```python
from build123d import *

# Parameters (mm, degrees)
BOSS_EXTRU_1_DEPTH           = 40
ENL_V_MAT_EXTRU_1_DEPTH      = 76.498344353
ENL_V_MAT_EXTRU_1_DEPTH_BACK = 76.498344353
ESQUISSE2_R                  = 2.25
ENL_V_MAT_EXTRU_2_DEPTH      = 76.498344353
ENL_V_MAT_EXTRU_2_DEPTH_BACK = 76.498344353
ESQUISSE3_R                  = 2.25
ENL_V_MAT_EXTRU_3_DEPTH      = 96.640449297
ENL_V_MAT_EXTRU_3_DEPTH_BACK = 20
ESQUISSE4_R                  = 2.1
BOSS_EXTRU_2_DEPTH           = 4
BOSS_EXTRU_3_START           = -40
BOSS_EXTRU_3_DEPTH           = 4
BOSS_EXTRU_4_DEPTH           = 3
BOSS_EXTRU_4_DEPTH_BACK      = 3
BOSS_EXTRU_4_START           = -20
CONG_1_R                     = 4


with BuildPart() as part:
    # Esquisse1 → Boss.-Extru.1 (new body)
    with BuildSketch(Plane(origin=(0, 0, 0), x_dir=(0, 0, -1), z_dir=(1, 0, 0))):
        Polygon((0, 0), (40, 0), (40, 10), (0, 10), (0, 36), (-15, 36), (-35, 1.358983849), (-20, -7.301270189), (-10, -7.301270189), (-10, -40), (0, -40), align=None)
    extrude(amount=BOSS_EXTRU_1_DEPTH)

    # Esquisse2 → Enlèv. mat.-Extru.1 (cut, two sides: drawn at the far end of the back side and taken through both)
    with BuildSketch(Plane(origin=(0, 10, 0), x_dir=(1, 0, 0), z_dir=(0, 1, 0)).offset(-ENL_V_MAT_EXTRU_1_DEPTH_BACK)):
        with Locations(Location((10, 30, 0), (0, 0, 270))):
            Circle(ESQUISSE2_R)
        with Locations(Location((30, 30, 0), (0, 0, 270))):
            Circle(ESQUISSE2_R)
        with Locations(Location((30, 10, 0), (0, 0, 270))):
            Circle(ESQUISSE2_R)
        with Locations(Location((10, 10, 0), (0, 0, 270))):
            Circle(ESQUISSE2_R)
    extrude(amount=ENL_V_MAT_EXTRU_1_DEPTH + ENL_V_MAT_EXTRU_1_DEPTH_BACK, mode=Mode.SUBTRACT)

    # Esquisse3 → Enlèv. mat.-Extru.2 (cut, two sides: drawn at the far end of the back side and taken through both)
    with BuildSketch(Plane.XY.offset(10).offset(-ENL_V_MAT_EXTRU_2_DEPTH_BACK)):
        with Locations((10, -33.650635095)):
            Circle(ESQUISSE3_R)
        with Locations((30, -33.650635095)):
            Circle(ESQUISSE3_R)
        with Locations((30, -13.650635095)):
            Circle(ESQUISSE3_R)
        with Locations((10, -13.650635095)):
            Circle(ESQUISSE3_R)
    extrude(amount=ENL_V_MAT_EXTRU_2_DEPTH + ENL_V_MAT_EXTRU_2_DEPTH_BACK, mode=Mode.SUBTRACT)

    # Esquisse4 → Enlèv. mat.-Extru.3 (cut, two sides: drawn at the far end of the back side and taken through both)
    with BuildSketch(Plane(origin=(0, 15.495190528, 26.838457268), x_dir=(1, 0, 0), z_dir=(0, 0.4999999999999946, 0.8660254037844419)).offset(-ENL_V_MAT_EXTRU_3_DEPTH_BACK)):
        with Locations(Location((20, 13.676914536, 0), (0, 0, 90))):
            Circle(ESQUISSE4_R)
        with Locations(Location((20, -6.323085464, 0), (0, 0, 90))):
            Circle(ESQUISSE4_R)
    extrude(amount=ENL_V_MAT_EXTRU_3_DEPTH + ENL_V_MAT_EXTRU_3_DEPTH_BACK, mode=Mode.SUBTRACT)

    # Esquisse5 → Boss.-Extru.2 (add)
    with BuildSketch(Plane(origin=(40, 0, 0), x_dir=(0, 0, -1), z_dir=(1, 0, 0))):
        Polygon((40, 10), (0, 36), (0, 10), align=None)
    extrude(amount=-BOSS_EXTRU_2_DEPTH)

    # Esquisse5<2> → Boss.-Extru.3 (add)
    with BuildSketch(Plane(origin=(40, 0, 0), x_dir=(0, 0, -1), z_dir=(1, 0, 0)).offset(BOSS_EXTRU_3_START)):
        Polygon((40, 10), (0, 36), (0, 10), align=None)
    extrude(amount=BOSS_EXTRU_3_DEPTH)

    # Esquisse5<3> → Boss.-Extru.4 (add, two sides: drawn at the far end of the back side and taken through both)
    with BuildSketch(Plane(origin=(40, 0, 0), x_dir=(0, 0, -1), z_dir=(1, 0, 0)).offset(BOSS_EXTRU_4_START - BOSS_EXTRU_4_DEPTH_BACK)):
        Polygon((40, 10), (0, 36), (0, 10), align=None)
    extrude(amount=BOSS_EXTRU_4_DEPTH + BOSS_EXTRU_4_DEPTH_BACK)

    # Congé1
    cong_1_edges = [part.edges().sort_by_distance(p)[0] for p in [
        (0, 5, -40),
        (40, 5, -40),
        (0, -40, 5),
        (40, -40, 5),
    ]]
    fillet(cong_1_edges, radius=CONG_1_R)


solid = part.part
```
Verification items for the finished model (mm, model axes). A direction names the side the tool comes from. Round coordinates to 2 decimals unless told otherwise and drop trailing zeros. Write each loop counter-clockwise with the first axis right and the second up, starting at its lowest first coordinate (ties: lowest second). Pieces come first, ordered by that corner, then holes. Notation, with made-up numbers: (18, -26.75) -> (67, -26.75) arc R26 ccw to (67, 4.25) -> close; hole circle Ø5 at (83.5, 65). An arc over 180 degrees is marked (long way). Write each question's results on one line, items separated by ' | '.
Q1. Sectioned sample at A-A, the plane z = -30. Record the boundary of the cut face in (x, y).
Derived:
outline: (0, 0) -> (7.75, 0) -> (7.75, 10) -> (4, 10) -> (4, 16.5) -> (0, 16.5) -> close; (12.25, 0) -> (27.75, 0) -> (27.75, 10) -> (23, 10) -> (23, 16.5) -> (17, 16.5) -> (17, 10) -> (12.25, 10) -> close; (32.25, 0) -> (40, 0) -> (40, 16.5) -> (36, 16.5) -> (36, 10) -> (32.25, 10) -> close
Q2. Sectioned sample at D-D, the plane y = -18.5. Record the boundary of the cut face in (x, z), and give its area (3 significant figures).
Derived:
outline: (0, 0) -> (40, 0) -> (40, 10) -> (0, 10) -> close | area: 400 mm²
Q3. Sectioned sample at C-C, the plane z = -2. Record the boundary of the cut face in (x, y), and give its area (3 significant figures).
Derived:
outline: (0, 0) -> (40, 0) -> (40, 34.7) -> (36, 34.7) -> (36, 10) -> (23, 10) -> (23, 34.7) -> (17, 34.7) -> (17, 10) -> (4, 10) -> (4, 34.7) -> (0, 34.7) -> close | area: 746 mm²
Q4. Thickness scan on probe 1 along Y at (x, z) = (10, 6); probe 2 along X at (y, z) = (3.25, -30); probe 3 along X at (y, z) = (-15, 8.5). Record the ranges inside material, lowest first.
Derived:
probe 1: y = -40 to -35.9, -31.4 to -15.9, -11.4 to 36 | probe 2: x = 0 to 7.75, 12.25 to 27.75, 32.25 to 40 | probe 3: x = 0 to 8.2, 11.8 to 28.2, 31.8 to 40
Q5. Access from +Z, -Z, +X, -X, +Y, -Y to the whole of each face (thin tool, end or side, straight path). Record for faces 1 (the face through (30.099, 4.93, -12.248)), 2 (the face through (29, 23, 0)), 3 (the face through (20, -23, 10)).
Derived:
face 1: +Y, -Y | face 2: -Z, +Y | face 3: +Z, +X, -X, -Y
Q6. Draft check along X on faces 4 (the face through (11.52, 4.93, -11.66)), 5 (the face through (0, 9, 0)), 6 (the face through (2, 23, -20)). Enter one of: released by +X, released by -X, zero draft, split by the parting line, or undercut.
Derived:
face 4: undercut | face 5: released by -X | face 6: zero draft
Q7. Go/stop test with flat-tipped pins: pin 1 Ø7 at (x, y) = (10, -13.65) entering from -Z; pin 2 Ø10 at (x, y) = (28, -3.5) entering from +Z; pin 3 Ø2 at (x, y) = (17, 3) entering from +Z; pin 4 Ø4 at (y, z) = (21, 5) entering from -X. Record where each tip stops, or that it passes through.
Derived:
pin 1: stops at z = 0 | pin 2: stops at z = 35 | pin 3: stops at z = 34.63 | pin 4: stops at x = 0
Q8. Sectioned sample at B-B, the plane x = 30. Record the boundary of the cut face in (y, z).
Derived:
outline: (-40, 0) -> (-35.9, 0) -> (-35.9, 10) -> (-40, 10) -> close; (-31.4, 0) -> (-15.9, 0) -> (-15.9, 10) -> (-31.4, 10) -> close; (-11.4, 0) -> (0, 0) -> (0, -7.75) -> (10, -7.75) -> (10, 0) -> (36, 0) -> (36, 15) -> (1.36, 35) -> (-7.3, 20) -> (-7.3, 10) -> (-11.4, 10) -> close; (0, -40) -> (10, -40) -> (10, -32.25) -> (0, -32.25) -> close; (0, -27.75) -> (10, -27.75) -> (10, -12.25) -> (0, -12.25) -> close
